The listing builds one solid part. Answer for the finished solid, in the listing's coordinates (mm). Face numbers are marked on the shaded views. Round coordinates to 2 decimals unless told otherwise and drop trailing zeros. Order: outer loops, then holes, each group sorted by start corner. A loop starts at its lowest first (then second) coordinate and runs counter-clockwise, first axis right, second up. Notation, with made-up numbers: (-37.75, 64) - (-20.75, 64) arc R25 ccw to (-20.75, 83) - close; hole circle Ø8 at (68, 68.5). An arc over 180 degrees is marked (long way). Use CSV: the item, a comma, the result in double quotes. Start each with the question number.
Item 1: Find section C-C, the plane y = -15.5. Give the vertices of the cut face in (x, z).
Item 2: Find section A-A, the plane y = -54.5. Give the vertices of the cut face in (x, z).
Item 3: Determine the mould class of the marked faces 1, 2 and 3 for opening direction Y: +Y half, -Y half, draft (parallel to the pull), parting line (faces both ways), or undercut.
Item 4: Find section D-D, the plane z = 2.75. Give the vertices of the cut face in (x, y), plus the area to 3 significant figures.
Item 5: Find section B-B, the plane x = -6.5. Give the vertices of the cut face in (y, z), plus the area to 3 significant figures.
Item 6: Straight lines are drawn through the part: line 1 along Y through (x, z) = (0, 7.5); line 2 along X through (y, z) = (-30, 2.5); line 3 along Y through (x, z) = (3, 3.75). For each, find the intervals that lie inside material, in ascending order. Write a range as [from, to].
Item 7: Flat-ended cylindrical pins translate along their axes: P1, Ø8, axis at x = 13, y = -36, coming from the -Z side; P2, Ø1.5, axis at y = -33.5, z = 5, coming from the -X side; P3, Ø3, axis at x = 27, y = -15.5, coming from the +Z side; P4, Ø4, axis at x = -4.5, y = -9.5, coming from the +Z side. Find the tip coordinate at first contact, or state that the pin passes through.
```python
from build123d import *

# Parameters (mm, degrees)
F1_DEPTH = 60
F2_R     = 21
F3_DEPTH = 25


with BuildPart() as f1:
    # F0 (on Front) → F1 (new body)
    with BuildSketch(Plane.XZ):
        with BuildLine():
            ThreePointArc((0, 11.266028276), (-18.3842554453, 8.3801171833), (-35, 0))
            Line((-35, 0), (0, 0))
            Line((0, 0), (0, 4.383014138))
            ThreePointArc((0, 4.383014138), (-1.25, 5.633014138), (0, 6.883014138))
            Line((0, 6.883014138), (0, 11.266028276))
        make_face()
        with BuildLine():
            Line((0, 0), (35, 0))
            ThreePointArc((35, 0), (18.3842554453, 8.3801171833), (0, 11.266028276))
            Line((0, 11.266028276), (0, 6.883014138))
            ThreePointArc((0, 6.883014138), (0.8838834765, 6.5168976145), (1.25, 5.633014138))
            ThreePointArc((1.25, 5.633014138), (0.8838834765, 4.7491306615), (0, 4.383014138))
            Line((0, 4.383014138), (0, 0))
        make_face()
    extrude(amount=F1_DEPTH)

    # F2 (on face) → F3 (cut)
    with BuildSketch(Plane(origin=(0, 0, 0), x_dir=(1, 0, 0), z_dir=(0, 0, -1))):
        with Locations((0, 30)):
            Circle(F2_R)
    extrude(amount=-F3_DEPTH, mode=Mode.SUBTRACT)


solid = f1.part
```
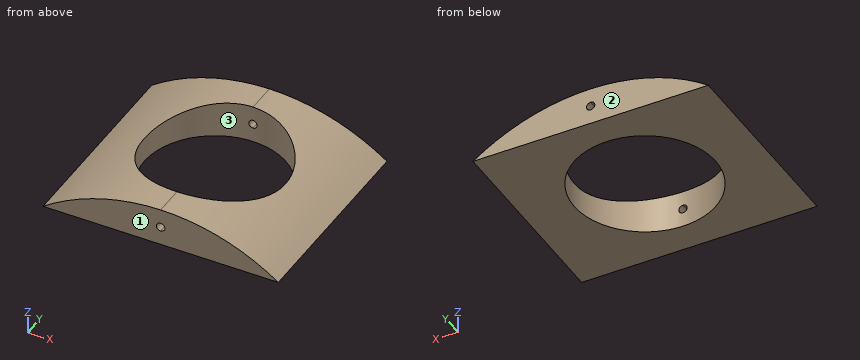
Worked out:
1,outline,"(-35, 0) - (-15.19, 0) - (-15.19, 9.31) arc R60 ccw to start; (15.19, 0) - (35, 0) arc R60 ccw to (15.19, 9.31) - close"
2,outline,"(-35, 0) - (35, 0) arc R60 ccw to start; hole circle Ø2.5 at (0, 5.63)"
3,face 1,"-Y half"
3,face 2,"+Y half"
3,face 3,"undercut"
4,outline,"(-30.81, -60) - (30.81, -60) - (30.81, 0) - (-30.81, 0) - close; hole circle Ø42 at (0, -30)"
4,area,"2,310 mm²"
5,outline,"(-60, 0) - (-49.97, 0) - (-49.97, 10.91) - (-60, 10.91) - close; (-10.03, 0) - (0, 0) - (0, 10.91) - (-10.03, 10.91) - close"
5,area,"219 mm²"
6,line 1,"y = [-60, -51], [-9, 0]"
6,line 2,"x = [-31.23, -21], [21, 31.23]"
6,line 3,"y = [-60, -50.78], [-9.22, 0]"
7,P1,"passes through"
7,P2,"stops at x = -28.15"
7,P3,"stops at z = 5.58"
7,P4,"stops at z = 11.21"
